Geometry check sheet. Reference: drawing and pictorial views, mm from the part's lowest x, y, z. A direction names the side the tool comes from. Give positions to 0.01 mm unless a question says otherwise; leave off trailing zeros. Order: outer loops, then holes, each group sorted by start corner. A loop starts at its lowest first (then second) coordinate and runs counter-clockwise, first axis right, second up.
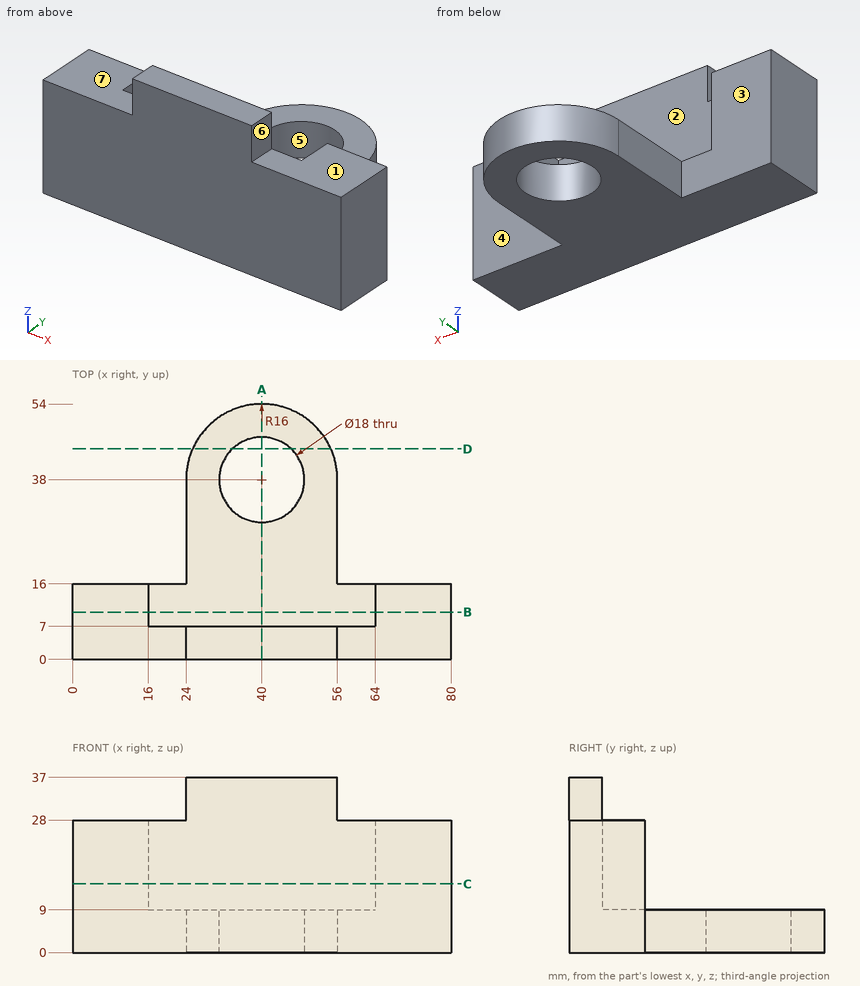
(1) Set-up check for the marked faces 1, 2, 3 and 4: record each of +Z, -Z, +X, -X, +Y, -Y from which the full face is reachable in a straight line by a thin tool's end or side.
Response values:
face 1: +Z, +X, +Y, -Y
face 2: +Z, +Y
face 3: +Z, -Z, -X, +Y
face 4: +Z, -Z, +X, +Y
(2) Cross-section at A-A on x = 40. Enter the section's corners in (y, z), then the cut area to 3 significant figures.
Response values:
outline: (0, 0) - (29, 0) - (29, 9) - (7, 9) - (7, 37) - (0, 37) - close; (47, 0) - (54, 0) - (54, 9) - (47, 9) - close
area: 520 mm2
(3) Cross-section at B-B on y = 10. Enter the section's corners in (x, z), then the cut area to 3 significant figures.
Response values:
outline: (0, 0) - (80, 0) - (80, 28) - (64, 28) - (64, 9) - (16, 9) - (16, 28) - (0, 28) - close
area: 1,330 mm2
(4) Cross-section at C-C on z = 14.5. Enter the section's corners in (x, y).
Response values:
outline: (0, 0) - (80, 0) - (80, 16) - (64, 16) - (64, 7) - (16, 7) - (16, 16) - (0, 16) - close
(5) Cross-section at D-D on y = 44.5. Enter the section's corners in (x, z).
Response values:
outline: (25.38, 0) - (33.78, 0) - (33.78, 9) - (25.38, 9) - close; (46.22, 0) - (54.62, 0) - (54.62, 9) - (46.22, 9) - close
(6) Material ranges on L1, parallel to Y at x = 40, z = 2; L2, parallel to Y at x = 16.5, z = 22; L3, parallel to Z at x = 18, y = 14, recorded low to high.
Response values:
L1: y = 0 to 29, 47 to 54
L2: y = 0 to 7
L3: z = 0 to 9
(7) Gauge pin test, flat ends, axial feed: pin 1 Ø7 at (y, z) = (27.5, 3.5) entering from -X; pin 2 Ø7.5 at (y, z) = (4, 33.5) entering from +X; pin 3 Ø11 at (x, y) = (40, 38) entering from -Z; pin 4 Ø12 at (x, z) = (8.5, 9.5) entering from +Y. Record the tip position at first contact, or that the pin passes through.
Response values:
pin 1: stops at x = 24
pin 2: stops at x = 56
pin 3: passes through
pin 4: stops at y = 16
(8) Release check for a two-part mould opening along X. For the marked faces 5, 6 and 7 record: released by +X, released by -X, zero draft, split by the parting line, or undercut.
Response values:
face 5: undercut
face 6: released by +X
face 7: zero draft
